Could you check a few things on this model? Use its own coordinates, in mm. A direction names the side the tool comes from. Give positions to 0.01 mm unless a question says otherwise; leave off trailing zeros. Order: outer loops, then holes, each group sorted by start corner. A loop starts at its lowest first (then second) coordinate and runs counter-clockwise, first axis right, second up. Notation, with made-up numbers: M 80,59 L 109,59 A17 ccw 109,71 Z; hole C 50,-10.75 d1. An arc over 180 degrees is marked long. Answer in a Markdown table with one row per item. Add a question column.
```python
from build123d import *

# Parameters (mm, degrees)
SKETCH1_R           = 35.00000000000001
BOSS_EXTRUDE1_DEPTH = 1000
CUT_EXTRUDE1_DEPTH  = 750
SKETCH22_R          = 30
CUT_EXTRUDE2_DEPTH  = 750
SKETCH23_W          = 366.89615803266116
SKETCH23_H          = 201.36798200180615
BOSS_EXTRUDE2_DEPTH = 500
CUT_EXTRUDE4_DEPTH  = 500
SKETCH26_W          = 450.22684379892416
SKETCH26_H          = 39.01754234256356
CUT_EXTRUDE5_DEPTH  = 500
BOSS_EXTRUDE3_REACH = 1516.531
SKETCH27_R          = 131.99999999999994
CUT_EXTRUDE8_DEPTH  = 1520.3228139489233


with BuildPart() as part:
    # Sketch1 → Boss-Extrude1 (new body)
    with BuildSketch(Plane.XY):
        Circle(SKETCH1_R)
    extrude(amount=BOSS_EXTRUDE1_DEPTH)

    # Sketch21 → Cut-Extrude1 (cut, symmetric)
    with BuildSketch(Plane(origin=(0, 0, 0), x_dir=(1, 0, 0), z_dir=(0, 1, 0))):
        with BuildLine():
            ThreePointArc((0, 0), (-24.748737341529168, -10.251262658470836), (-35.00000000000001, -35.00000000000001))
            Line((-35.00000000000001, -35.00000000000001), (-35.00000000000001, 14.56189922191023))
            Line((-35.00000000000001, 14.56189922191023), (35.00000000000001, 14.56189922191023))
            Line((35.00000000000001, 14.56189922191023), (35.00000000000001, -35.000000000000085))
            ThreePointArc((35.00000000000001, -35.000000000000085), (24.748737341529196, -10.251262658470868), (0, 0))
        make_face()
    extrude(amount=CUT_EXTRUDE1_DEPTH, both=True, mode=Mode.SUBTRACT)

    # Sketch22 → Cut-Extrude2 (cut, symmetric)
    with BuildSketch(Plane(origin=(0, 0, 0), x_dir=(1, 0, 0), z_dir=(0, 1, 0))):
        with Locations(Location((0, -34.999999999999964, 0), (0, 0, 270))):
            Circle(SKETCH22_R)
    extrude(amount=CUT_EXTRUDE2_DEPTH, both=True, mode=Mode.SUBTRACT)

    # Sketch23 → Boss-Extrude2 (add)
    with BuildSketch(Plane.XY.offset(1000)):
        Rectangle(SKETCH23_W, SKETCH23_H)
    extrude(amount=BOSS_EXTRUDE2_DEPTH)

    # Sketch24 → Cut-Extrude4 (cut)
    with BuildSketch(Plane.XZ.offset(100.68399100090306)):
        Polygon((79.59360487116518, 1500), (-78.45567005550114, 1500), (-78.45567005550113, 1058.1623604619979), (-34.99999999999988, 1024.8865781005384), (36.137934815664146, 1024.8865781005381), (79.59360487116518, 1058.1623604619977), align=None)
        Polygon((-100, 1049.7731562010758), (-100, 1500), (-183.44807901633058, 1500), (-183.44807901633058, 1000), (-35, 1000), align=None)
        Polygon((100, 1049.7731562010758), (35.00000000000001, 1000), (183.44807901633058, 1000), (183.44807901633058, 1500), (100, 1500), align=None)
    extrude(amount=-CUT_EXTRUDE4_DEPTH, mode=Mode.SUBTRACT)

    # Sketch26 → Cut-Extrude5 (cut)
    with BuildSketch(Plane.ZY.offset(100)):
        with Locations((1274.886578100538, 81.1752198296213)):
            Rectangle(SKETCH26_W, SKETCH26_H)
        Polygon((1000, 61.66644865833952), (1049.7731562010758, 61.66644865833952), (1049.7731562010758, 100.68399100090308), (1024.8865781005381, 100.68399100090308), (1000, 100.68399100090308), align=None)
        Polygon((1500, -100.68399100090306), (1500, -61.666448658339505), (1049.7731562010758, -61.666448658339505), (1049.7731562010758, -100.68399100090305), align=None)
        Polygon((1049.7731562010758, -100.68399100090305), (1049.7731562010758, -61.66644865833949), (1000, -61.666448658339505), (1000, -100.68399100090306), align=None)
    extrude(amount=-CUT_EXTRUDE5_DEPTH, mode=Mode.SUBTRACT)

    # Boss-Extrude3: up to this face of the body (flat: up to its plane)
    boss_extrude3_end = Plane(part.part.faces().sort_by_distance((100, 0, 1274.886578101))[0])
    # Sketch27 → Boss-Extrude3 (add, up to the picked face)
    with BuildSketch(Plane.ZY.offset(100), mode=Mode.PRIVATE) as boss_extrude3_sk1:
        with Locations((1368, -3.431949648798167)):
            Circle(SKETCH27_R)
    boss_extrude3_tool1 = split(extrude(boss_extrude3_sk1.sketch, amount=-BOSS_EXTRUDE3_REACH, mode=Mode.PRIVATE), bisect_by=boss_extrude3_end, keep=Keep.BOTH, mode=Mode.PRIVATE)
    add(boss_extrude3_tool1.solids().sort_by(Axis((-100, -3.43195, 1368), (1, 0, 0)))[0])

    # Sketch28 → Cut-Extrude8 (cut, through all)
    with BuildSketch(Plane.ZY.offset(100)):
        with BuildLine():
            Line((1576.6741063083334, 113.68167915660561), (1386.7378452368366, 127.23133194125066))
            ThreePointArc((1386.7378452368366, 127.2313319412505), (1442.39663439627, 105.60538703230257), (1482.8311740680433, 61.66644865833952))
            Line((1482.8311740680433, 61.66644865833952), (1500, 61.66644865833952))
            Line((1500, 61.66644865833953), (1500, -3.4319477522261153))
            Line((1500, -3.4319477522261153), (1500, -61.666448658339505))
            Line((1500, -61.666448658339505), (1486.4598798121447, -61.666448658339505))
            ThreePointArc((1486.4598798121447, -61.666448658339476), (1437.7748025104354, -115.48317425000337), (1368, -135.43194964879822))
            Line((1368, -135.4319496487982), (1367.9999999999998, -201.07935807583712))
            Line((1367.9999999999998, -201.07935807583712), (1604.9218917009885, -125.07936404321737))
            Line((1604.9218917009885, -125.07936404321737), (1576.6741063083334, 113.68167915660561))
        make_face()
        with BuildLine():
            Line((1500, -61.666448658339505), (1500, -3.4319477522261153))
            ThreePointArc((1500, -3.431947752226116), (1496.5704169816079, -33.32589346983822), (1486.4598798121447, -61.666448658339476))
            Line((1486.4598798121447, -61.666448658339505), (1500, -61.666448658339505))
        make_face()
        with BuildLine():
            Line((1500, 61.66644865833952), (1482.8311740680433, 61.66644865833952))
            ThreePointArc((1482.8311740680433, 61.66644865833952), (1495.63564324576, 30.23023348362874), (1500, -3.431947752226116))
            Line((1500, -3.4319477522261153), (1500, 61.66644865833953))
        make_face()
    extrude(amount=-CUT_EXTRUDE8_DEPTH, mode=Mode.SUBTRACT)


solid = part.part
```
1. Suppose I cut it at B-B on x = 54. List the corners of the cut face in (y, z) for me.
2. Will these pins go through, and if not, where does the flat tip stop? P1, Ø4, axis at x = 75.5, y = 1, coming from the +Z side; P2, Ø5, axis at x = -47, y = 21, coming from the -Z side; P3, Ø1, axis at x = -54, y = 86, coming from the -Z side.
3. For faces 4 (the flat face through (-57.032, -0.863, 1041.757)), 5 (the cylindrical face through (-7.587, -34.168, 493)), 6 (the flat face through (-82, -61.666, 1107)), 7 (the flat face through (81, 61.666, 1098)), 8 (the flat face through (100, -2, 1278)), which set-ups out of +Z, -Z, +X, -X, +Y, -Y let a thin tool reach every point of the face, with its end or its side?
4. Suppose I cut it at A-A on z = 1152. List the corners of the cut face in (x, y) for me, plus the area to 3 significant figures.
5. If I drill on line 1 along Z through (x, y) = (0, 4); line 2 along Z through (x, y) = (0, -6.5); line 3 along X through (y, z) = (-4, 35), over which ranges is the centre line in solid material (lowest first)? Write a range as [from, to].
6. Thinking about a two-plate mould opening in X: for faces 1 (the cylindrical face through (0.77, 0.49, 0.01)), 2 (the flat face through (67.95, -0.86, 1025.23)), 3 (the flat face through (0, -1, 1024.887)), which applies, pulls with the +X half, pulls with the -X half, needs draft (parallel to the pull), parting line crosses it, or undercut?
7. Suppose I cut it at D-D on z = 495.5. List the corners of the cut face in (x, y) for me.
8. Suppose I cut it at C-C on x = 0. List the corners of the cut face in (y, z) for me.
Findings below:
| question | item | result |
|---|---|---|
| 1 | outline | C -3.43,1368 d264; M -61.67,1014.55 L 61.67,1014.55 L 61.67,1038.56 L -61.67,1038.56 Z |
| 2 | P1 | z = 1499.98 |
| 2 | P2 | z = 1007.27 |
| 2 | P3 | z = 1270.45 |
| 3 | face 4 | +Y, -Y |
| 3 | face 5 | -Z |
| 3 | face 6 | -Z, +X, -X, -Y |
| 3 | face 7 | -Z, +X, -X, +Y |
| 3 | face 8 | +Z, -Z, +X, +Y, -Y |
| 4 | outline | M -100,-61.67 L -78.46,-61.67 L -78.46,61.67 L -100,61.67 Z; M 79.59,-61.67 L 100,-61.67 L 100,61.67 L 79.59,61.67 Z |
| 4 | area | 5,170 mm2 |
| 5 | line 1 | [0, 5], [65, 1024.89], [1236.21, 1499.79] |
| 5 | line 2 | [0, 5], [65, 1024.89], [1236.04, 1499.96] |
| 5 | line 3 | [-34.77, -30], [30, 34.77] |
| 6 | face 1 | parting line crosses it |
| 6 | face 2 | pulls with the +X half |
| 6 | face 3 | undercut |
| 7 | outline | C 0,0 d70 |
| 8 | outline | C -3.43,1368 d264; M -61.67,1000 L -35,1000 L -35,65 L 35,65 L 35,1000 L 61.67,1000 L 61.67,1024.89 L -61.67,1024.89 Z; M -35,0 L 35,0 L 35,5 L -35,5 Z |
